Can you work these out from the model? Positions are in its coordinate system, mm. Face numbers are marked on the shaded views. A direction names the side the tool comes from. Coordinates: 2 decimals unless noted, no trailing zeros. Order: outer loops, then holes, each group sorted by start corner. A loop starts at its lowest first (then second) coordinate and runs counter-clockwise, first axis right, second up. Notation, with made-up numbers: (32.25, 49.25) - (63.25, 49.25) arc R12 ccw to (63.25, 68.25) - close; hole circle Ø9 at (32, -23.5). An arc over 180 degrees is marked (long way). Return JSON: item names as keys, results as strings. Group by question number.
1) For pin 1 Ø5 at (x, y) = (-3, 7.5) entering from +Z; pin 2 Ø7.5 at (x, z) = (0, 14) entering from -Y; pin 3 Ø6 at (x, z) = (0, 12.9) entering from +Y, each with a flat end and sliding along its axis, tell me the tip position at first contact or that it passes through.
2) Imagine slicing it at A-A (y = -10). Write out the boundary of the cut face in (x, z) (3 decimals), and give its area (3 significant figures).
3) Which directions (+Z, -Z, +X, -X, +Y, -Y) give clear straight access to the entire face, cutting with the end or side of a thin tool? Please do the marked faces 1 and 2.
4) Imagine slicing it at D-D (y = 1.5). Write out the boundary of the cut face in (x, z).
5) If I drill on line 1 along Y through (x, z) = (-0.5, 21); line 2 along Y through (x, z) = (-5.5, 19.75); line 3 along X through (y, z) = (4.5, 20.25), over which ranges is the centre line in solid material (lowest first)?
6) Imagine slicing it at C-C (x = -1.5). Give the number of separate pieces and of enclosed holes in the cut face, and give its area (3 significant figures).
7) If we mould it in two halves opening along X, with no side actions, what happens to the marked faces 3, 4 and 5? For each: pulls with the +X half, pulls with the -X half, needs draft (parallel to the pull), parting line crosses it, or undercut.
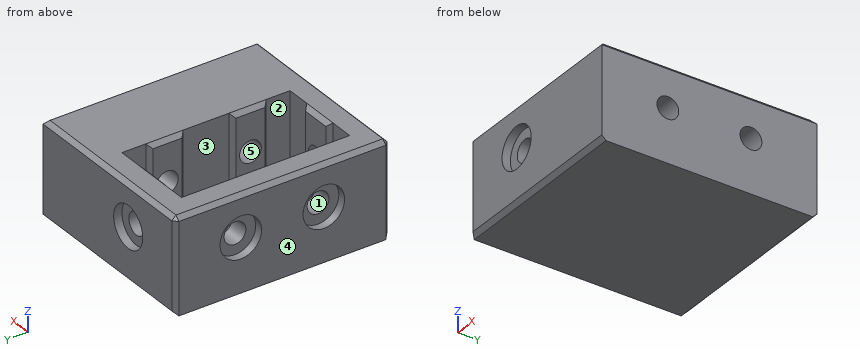
Autodesk Fusion 360 part; units mm, degrees
sketch "Main Profile" plane through (0, 0, 0) normal (0, 0, 1) x (1, 0, 0)
  line L0 (10.25, -20.25) -> (-10.25, -20.25)
  line L1 (-10.25, -20.25) -> (-10.25, 20.25)
  line L2 (-10.25, 20.25) -> (10.25, 20.25)
  line L3 (10.25, 20.25) -> (10.25, -20.25)
  line L4 (10.25, -20.25) -> (-10.25, 20.25) construction
  line L5 (-10.25, -20.25) -> (10.25, 20.25) construction
  line L6 (-16, -25.9) -> (16, -25.9)
  line L7 (16, -25.9) -> (16, 25.9)
  line L8 (16, 25.9) -> (-16, 25.9)
  line L9 (-16, 25.9) -> (-16, -25.9)
  line L10 (-16, -25.9) -> (16, 25.9) construction
  line L11 (16, -25.9) -> (-16, 25.9) construction
  line L12 (-3.5, 19.25) -> (3.5, 19.25)
  line L13 (3.5, 19.25) -> (4.5, 20.25)
  line L14 (-3.5, 19.25) -> (-4.5, 20.25)
  line L15 (0, 20.25) -> (0, 19.25) construction
  line L16 (-9.25, 6.5) -> (-9.25, 13.5)
  line L17 (-9.25, 13.5) -> (-10.25, 14.5)
  line L18 (-9.25, 6.5) -> (-10.25, 5.5)
  line L19 (9.25, 13.5) -> (9.25, 6.5)
  line L20 (9.25, 6.5) -> (10.25, 5.5)
  line L21 (9.25, 13.5) -> (10.25, 14.5)
  line L22 (9.25, -13.5) -> (10.25, -14.5)
  line L23 (9.25, -6.5) -> (9.25, -13.5)
  line L24 (9.25, -6.5) -> (10.25, -5.5)
  line L25 (3.5, -19.25) -> (4.5, -20.25)
  line L26 (3.5, -19.25) -> (-3.5, -19.25)
  line L27 (-3.5, -19.25) -> (-4.5, -20.25)
  line L28 (-9.25, -13.5) -> (-10.25, -14.5)
  line L29 (-9.25, -13.5) -> (-9.25, -6.5)
  line L30 (-9.25, -6.5) -> (-10.25, -5.5)
  point P0 (0, 10)
  dimension "d1" = 40.5
  dimension "d2" = 20.5
  dimension "d3" = 32
  dimension "d4" = 51.8
  dimension "d5" = 1
  dimension "d6" = 135
  dimension "d7" = 7
  dimension "d8" = 135
  dimension "d9" = 10.25
  dimension "d11" = 360
  dimension "d13" = 360
extrude "Extrude1" add sketch "Main Profile" along normal blind 3 contours L0 L1 L2 L3 L12 L13 L14 L16 L17 L18 L19 L20 L21 L22 L23 L24 L25 L26 L27 L28 L29 L30 | L0 L25 L26 L27 | L3 L22 L23 L24 | L3 L19 L20 L21 | L1 L28 L29 L30 | L1 L16 L17 L18 | L2 L12 L13 L14 | L6 L7 L8 L9
extrude "Extrude2" add sketch "Main Profile" along normal blind 22.9 contours L0 L25 L26 L27 | L3 L22 L23 L24 | L3 L19 L20 L21 | L1 L28 L29 L30 | L1 L16 L17 L18 | L2 L12 L13 L14 | L6 L7 L8 L9
sketch "Short Side" plane through (0, 25.9, 0) normal (0, 1, 0) x (-1, 0, 0)
  line L0 (-16, 0) -> (16, 0)
  line L1 (16, 0) -> (16, 22.9)
  line L2 (16, 22.9) -> (-16, 22.9)
  line L3 (-16, 22.9) -> (-16, 0)
  circle A0 centre (0, 12.9) radius 5
  circle A1 centre (0, 12.9) radius 2.625
  dimension "d18" = 10
  dimension "d19" = 5.25
  dimension "d20" = 12.9
extrude "Extrude3" cut sketch "Short Side" against normal blind 63.819 contours A1
extrude "Extrude4" cut sketch "Short Side" against normal blind 2 contours A0
extrude "Extrude5" cut sketch "Short Side" along normal blind 2 from surface at -51.8 contours A0
sketch "Long Side" plane through (-16, 0, 0) normal (-1, 0, 0) x (0, -1, 0)
  line L0 (-25.9, 0) -> (25.9, 0)
  line L1 (25.9, 0) -> (25.9, 22.9)
  line L2 (25.9, 22.9) -> (-25.9, 22.9)
  line L3 (-25.9, 22.9) -> (-25.9, 0)
  circle A0 centre (-10, 12.9) radius 5
  circle A1 centre (-10, 12.9) radius 2.625
  circle A2 centre (10, 12.9) radius 5
  circle A3 centre (10, 12.9) radius 2.625
  dimension "d28" = 10
  dimension "d29" = 5.25
  dimension "d30" = 10
  dimension "d31" = 12.9
  dimension "d34" = 20
  dimension "d35" = 0
extrude "Extrude6" cut sketch "Long Side" against normal blind 62.946 contours A1 | A3
extrude "Extrude7" cut sketch "Long Side" against normal blind 2 contours A0 | A2
move_face "OffsetFaces1" offset 13.3 1 faces at (16, -21.4652, 11.8029)
chamfer "Chamfer1" distance 1 angle 45 14 edges at (9.25, 10, 22.9) (9.25, -10, 22.9) (-9.25, -10, 22.9) (0, -19.25, 22.9) (-9.25, 10, 22.9) (0, 19.25, 22.9) (6.65, 25.9, 22.9) (29.3, 0, 22.9) (6.65, -25.9, 22.9) (-16, 0, 22.9) (-16, -25.9, 11.45) (-16, 25.9, 11.45) (6.65, -25.9, 0) (6.65, 25.9, 0)
Calculated:
{
 "1": {"pin 1": "z = 3", "pin 2": "y = -23.9", "pin 3": "y = 23.9"},
 "2": {"outline": "(-16, 0) - (29.3, 0) - (29.3, 10.275) - (9.25, 10.275) - (9.25, 3) - (-9.25, 3) - (-9.25, 10.275) - (-14, 10.275) - (-14, 7.9) - (-16, 7.9) - close; (-16, 17.9) - (-14, 17.9) - (-14, 15.525) - (-9.25, 15.525) - (-9.25, 21.9) - (-10.25, 22.9) - (-15, 22.9) - (-16, 21.9) - close; (9.25, 15.525) - (29.3, 15.525) - (29.3, 21.9) - (28.3, 22.9) - (10.25, 22.9) - (9.25, 21.9) - close", "area": "517 mm2"},
 "3": {"face 1": "+X, -X", "face 2": "+Z"},
 "4": {"outline": "(-16, 0) - (29.3, 0) - (29.3, 21.9) - (28.3, 22.9) - (10.25, 22.9) - (10.25, 3) - (-10.25, 3) - (-10.25, 22.9) - (-15, 22.9) - (-16, 21.9) - close"},
 "5": {"line 1": "-25.9 to -19.25, 19.25 to 25.9", "line 2": "-25.9 to -20.25, 20.25 to 25.9", "line 3": "-16 to -10.25, 10.25 to 29.3"},
 "6": {"separate pieces": "3", "enclosed holes": "0", "area": "339 mm2"},
 "7": {"face 3": "undercut", "face 4": "pulls with the -X half", "face 5": "needs draft"}
}
